The listing builds one solid part. Answer for the finished solid, in the listing's coordinates (mm). Face numbers are marked on the shaded views. A direction names the side the tool comes from. Coordinates: 2 decimals unless noted, no trailing zeros. Loops run counter-clockwise (first coordinate to the right, second up) from the corner with the lowest first, then second, coordinate; pieces in that order, holes last. Notation, with made-up numbers: M -34.5,36 L -10.5,36 A18 ccw -10.5,43 Z; hole C 34.25,-6 d10. An arc over 180 degrees is marked long. Return JSON: item names as keys, results as strings. Group by question number.
1. Which of the six approach directions +Z, -Z, +X, -X, +Y, -Y give full straight-line access (tool end or side, diameter ignored) to the marked faces 1 and 2?
2. Section C-C (z = -5.5) is taken. Write down the section's boundary in (x, y).
3. The mould has two halves that part along Y. Classify the marked faces 3, 4 and 5: pulls with the +Y half, pulls with the -Y half, needs draft (parallel to the pull), parting line crosses it, or undercut.
4. Given P1, Ø8, axis at x = 8.5, y = -16, coming from the +Z side; P2, Ø8, axis at y = 0, z = -25, coming from the -X side; P3, Ø12, axis at x = 23, z = 23.5, coming from the -Y side; P4, Ø8, axis at y = 19, z = -2, coming from the -X side, each flat-ended and moving along its own axis, determine where each tip first touches the part or whether it passes through.
5. Section D-D (x = 22) is taken. Write down the section's boundary in (y, z), then the cut area to 3 significant figures.
6. Section A-A (y = 0) is taken. Write down the section's boundary in (x, z), then the cut area to 3 significant figures.
7. Straight lines are drawn through the part: L1, parallel to X at y = 0, z = -12; L2, parallel to Z at x = 22, y = 20. For each, find the intervals that lie inside material, in ascending order. Write a range as from..to.
```python
from build123d import *

# Parameters (mm, degrees)
SKETCH_R      = 30
SKETCH_R_2    = 21
PAD_DEPTH     = 4
SKETCH001_R   = 25
SKETCH001_R_2 = 21
PAD001_DEPTH  = 36
SKETCH002_R   = 25
SKETCH002_R_2 = 21
PAD002_DEPTH  = 30


with BuildPart() as part:
    # Sketch → Pad (new body)
    with BuildSketch(Plane.XY):
        Circle(SKETCH_R)
        Circle(SKETCH_R_2, mode=Mode.SUBTRACT)
    extrude(amount=PAD_DEPTH)

    # Sketch001 (on Face3 of Pad) → Pad001 (join)
    with BuildSketch(Plane(origin=(0, 0, 0), x_dir=(1, 0, 0), z_dir=(0, 0, -1))):
        Circle(SKETCH001_R)
        Circle(SKETCH001_R_2, mode=Mode.SUBTRACT)
    extrude(amount=PAD001_DEPTH)

    # Sketch002 (on Face3 of Pad001) → Pad002 (join)
    with BuildSketch(Plane.XY.offset(4)):
        Circle(SKETCH002_R)
        Circle(SKETCH002_R_2, mode=Mode.SUBTRACT)
    extrude(amount=PAD002_DEPTH)


solid = part.part
```
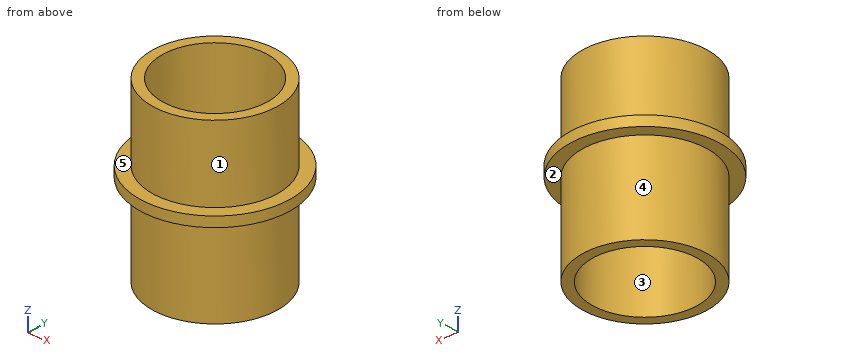
Worked out:
{
 "1": {"face 1": "+Z", "face 2": "-Z"},
 "2": {"outline": "C 0,0 d50; hole C 0,0 d42"},
 "3": {"face 3": "undercut", "face 4": "parting line crosses it", "face 5": "needs draft"},
 "4": {"P1": "z = 34", "P2": "x = -25", "P3": "y = -18.33", "P4": "x = -25.66"},
 "5": {"outline": "M -20.4,0 L -11.87,0 L -11.87,-36 L 11.87,-36 L 11.87,0 L 20.4,0 L 20.4,4 L 11.87,4 L 11.87,34 L -11.87,34 L -11.87,4 L -20.4,4 Z", "area": "1,730 mm^2"},
 "6": {"outline": "M -30,0 L -25,0 L -25,-36 L -21,-36 L -21,34 L -25,34 L -25,4 L -30,4 Z; M 21,-36 L 25,-36 L 25,0 L 30,0 L 30,4 L 25,4 L 25,34 L 21,34 Z", "area": "600 mm^2"},
 "7": {"L1": "-25..-21, 21..25", "L2": "0..4"}
}
